Verification items for this drawing (mm, ordinates from the low corner). A direction names the side the tool comes from. Give positions to 0.01 mm unless a question says otherwise; leave off trailing zeros. Loops run counter-clockwise (first coordinate to the right, second up) from the corner with the lowest first, then second, coordinate; pieces in that order, holes last. Notation, with made-up numbers: M 49,63 L 60,63 A9 ccw 60,80 Z; hole C 36.5,5 d10. An arc over 180 degrees is marked long. Answer in a Markdown table with one row per item.
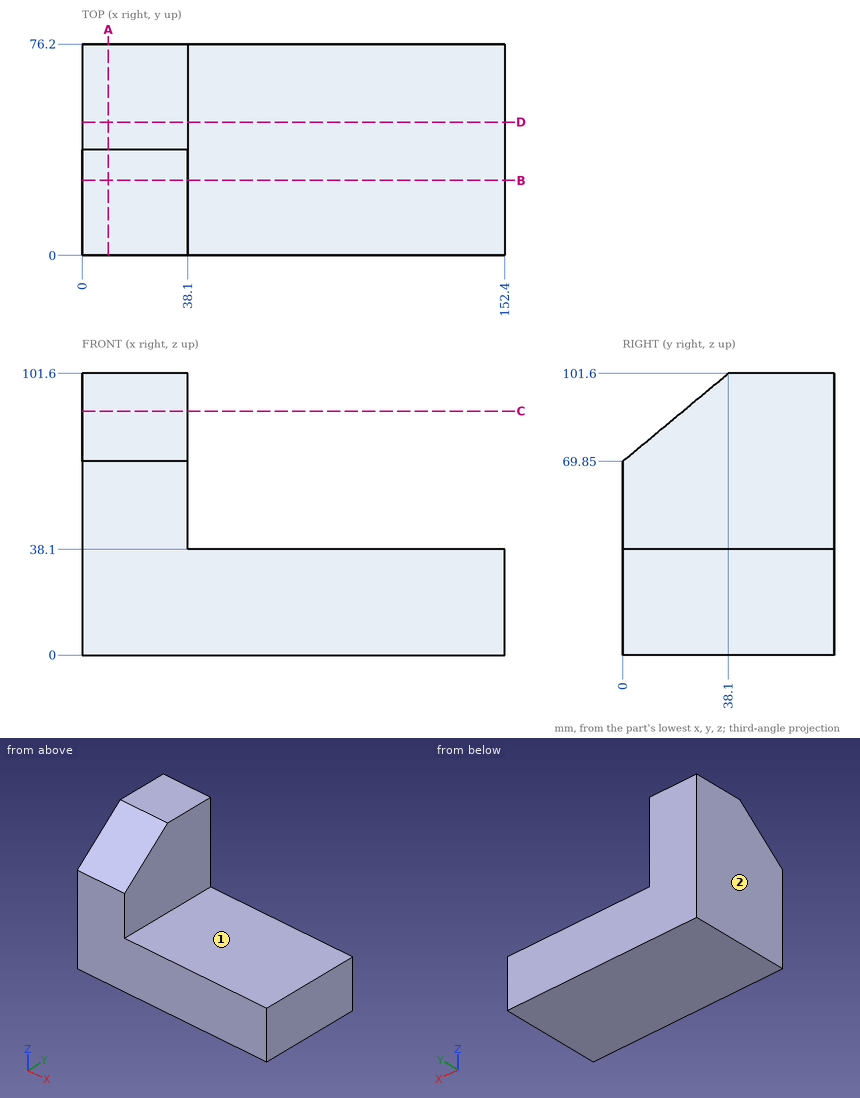
Item 1: Sectioned sample at C-C (z = 88). Record the cut outline in (x, y), and give its area (3 significant figures).
Reported:
| item | result |
|---|---|
| outline | M 0,21.78 L 38.1,21.78 L 38.1,76.2 L 0,76.2 Z |
| area | 2,070 mm^2 |
Item 2: Sectioned sample at A-A (x = 9.5). Record the cut outline in (y, z).
Reported:
| item | result |
|---|---|
| outline | M 0,0 L 76.2,0 L 76.2,101.6 L 38.1,101.6 L 0,69.85 Z |
Item 3: Scan lines: L1, parallel to Z at x = 42.5, y = 38; L2, parallel to Y at x = 35, z = 79. Record each from-to range of solid material in increasing order. Write a range as [from, to].
Reported:
| item | result |
|---|---|
| L1 | z = [0, 38.1] |
| L2 | y = [10.98, 76.2] |
Item 4: Sectioned sample at D-D (y = 48). Record the cut outline in (x, z), and give its area (3 significant figures).
Reported:
| item | result |
|---|---|
| outline | M 0,0 L 152.4,0 L 152.4,38.1 L 38.1,38.1 L 38.1,101.6 L 0,101.6 Z |
| area | 8,230 mm^2 |
Item 5: Sectioned sample at B-B (y = 27). Record the cut outline in (x, z).
Reported:
| item | result |
|---|---|
| outline | M 0,0 L 152.4,0 L 152.4,38.1 L 38.1,38.1 L 38.1,92.35 L 0,92.35 Z |
Item 6: Tool access check on the marked faces 1 and 2. Record the directions out of +Z, -Z, +X, -X, +Y, -Y that give a thin tool (end or side, any length) a straight path to the whole face; none if there is none.
Reported:
| item | result |
|---|---|
| face 1 | +Z, +X, +Y, -Y |
| face 2 | +Z, -Z, -X, +Y, -Y |
Item 7: Go/stop test with flat-tipped pins: pin 1 (10 mm diameter, centred on y = 12, z = 73, fed in from -X); pin 2 (3 mm diameter, centred on y = 40.5, z = 68, fed in from +X); pin 3 (5 mm diameter, centred on x = 47, y = 20, fed in from +Z). Record where each tip stops, or that it passes through.
Reported:
| item | result |
|---|---|
| pin 1 | stops at x = 0 |
| pin 2 | stops at x = 38.1 |
| pin 3 | stops at z = 38.1 |
